Input: part model. Units: mm. Frame: model coordinates. A direction names the side the tool comes from. Give positions to 0.01 mm unless a question says otherwise; leave off trailing zeros. Order: outer loops, then holes, each group sorted by start corner. A loop starts at its lowest first (then second) coordinate and runs counter-clockwise, first axis right, second up. Notation, with made-up numbers: (9, -29.5) - (38, -29.5) arc R15 cw to (38, -24.5) - close; hole circle Ø6 at (66.5, 20). An arc over 180 degrees is marked (long way). Answer in a Markdown table with one row per item. Add a question column.
from build123d import *

# Parameters (mm, degrees)
F0_W     = 12.7
F0_H     = 12.7
F1_DEPTH = 12.7
F2_R     = 1.5875
F3_DEPTH = 3.175
F4_W     = 12.7
F4_H     = 5.08
F5_DEPTH = 3.81
F6_W     = 12.7
F6_H     = 5.08
F7_DEPTH = 3.81


with BuildPart() as f1:
    # F0 (on Top) → F1 (new body)
    with BuildSketch(Plane.XY):
        with Locations((6.35, 6.35)):
            Rectangle(F0_W, F0_H)
    extrude(amount=F1_DEPTH)

    # F2 (on face) → F3 (join)
    with BuildSketch(Plane.XY.offset(12.7)):
        with Locations((6.35, 6.35)):
            Circle(F2_R)
    extrude(amount=F3_DEPTH)

    # F4 (on face) → F5 (join)
    with BuildSketch(Plane.XZ):
        with Locations((6.35, 6.35)):
            Rectangle(F4_W, F4_H)
    extrude(amount=F5_DEPTH)

    # F6 (on face) → F7 (join)
    with BuildSketch(Plane(origin=(0, 12.7, 0), x_dir=(-1, 0, 0), z_dir=(0, 1, 0))):
        with Locations((-6.35, 6.35)):
            Rectangle(F6_W, F6_H)
    extrude(amount=F7_DEPTH)


solid = f1.part
Q1. Section D-D, the plane z = 9.75. Return loops of the section in (x, y), then the cut area to 3 significant figures.
Q2. Section B-B, the plane y = 6.35. Return loops of the section in (x, z) (1 decimal).
Q3. Section A-A, the plane x = 6.35. Return loops of the section in (y, z) (1 decimal).
Q4. Access query for faces 1 (the flat face through (6, 15, 8.89)), 2 (the flat face through (6, 12.7, 2)), 3 (the flat face through (6, -2, 3.81)). Directions: +Z, -Z, +X, -X, +Y, -Y. A direction counts if a zero-diameter tool reaches every point of the face in a straight line with its end or side. Return the directions, or none.
Q5. Contact query for flat-ended pins moving along their axis: P1, Ø1.9, axis at x = 7, y = -2, coming from the +Z side; P2, Ø3, axis at x = 3.5, z = 2, coming from the +Y side; P3, Ø4, axis at x = 5, z = 11.5, coming from the -Y side. Output: stop coordinate, or through.
Q6. Line query: probe 1 along Z at (x, y) = (10, -1.5); probe 2 along Z at (x, y) = (3.75, 1.5). Output: solid intervals per line, ascending.
Q7. Section C-C, the plane x = 10.75. Return loops of the section in (y, z), then the cut area to 3 significant figures.
Computed:
| question | item | result |
|---|---|---|
| 1 | outline | (0, 0) - (12.7, 0) - (12.7, 12.7) - (0, 12.7) - close |
| 1 | area | 161 mm^2 |
| 2 | outline | (0, 0) - (12.7, 0) - (12.7, 12.7) - (7.9, 12.7) - (7.9, 15.9) - (4.8, 15.9) - (4.8, 12.7) - (0, 12.7) - close |
| 3 | outline | (-3.8, 3.8) - (0, 3.8) - (0, 0) - (12.7, 0) - (12.7, 3.8) - (16.5, 3.8) - (16.5, 8.9) - (12.7, 8.9) - (12.7, 12.7) - (7.9, 12.7) - (7.9, 15.9) - (4.8, 15.9) - (4.8, 12.7) - (0, 12.7) - (0, 8.9) - (-3.8, 8.9) - close |
| 4 | face 1 | +Z, +X, -X, +Y |
| 4 | face 2 | -Z, +X, -X, +Y |
| 4 | face 3 | -Z, +X, -X, -Y |
| 5 | P1 | stops at z = 8.89 |
| 5 | P2 | stops at y = 12.7 |
| 5 | P3 | stops at y = 0 |
| 6 | probe 1 | z = 3.81 to 8.89 |
| 6 | probe 2 | z = 0 to 12.7 |
| 7 | outline | (-3.81, 3.81) - (0, 3.81) - (0, 0) - (12.7, 0) - (12.7, 3.81) - (16.51, 3.81) - (16.51, 8.89) - (12.7, 8.89) - (12.7, 12.7) - (0, 12.7) - (0, 8.89) - (-3.81, 8.89) - close |
| 7 | area | 200 mm^2 |
